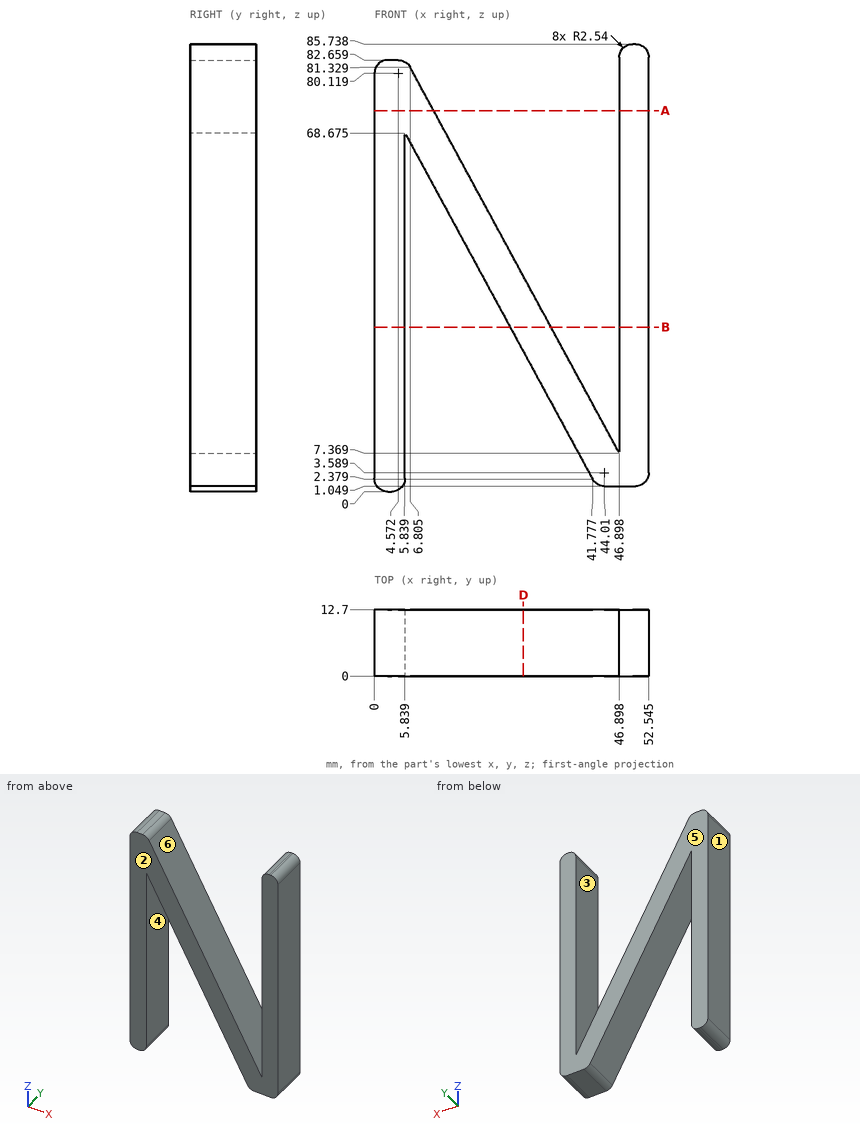
Check sheet for the drawn part. Datum: minimum x, y, z corner. Units: mm. A direction names the side the tool comes from. Coordinates: 2 decimals unless noted, no trailing zeros. Order: outer loops, then holes, each group sorted by start corner. A loop starts at its lowest first (then second) coordinate and runs counter-clockwise, first axis right, second up. Notation, with made-up numbers: (-14.75, 30.5) -> (37.25, 30.5) arc R31 ccw to (37.25, 63.5) -> close; hole circle Ø11 at (18.5, -31.75). An arc over 180 degrees is marked (long way). Write each question's results on one line, items separated by ' | '. Start each with the question number.
1) Material ranges on line 1 along X through (y, z) = (10.5, 45.5) (1 decimal); line 2 along X through (y, z) = (7, 15.5) (1 decimal); line 3 along X through (y, z) = (9.25, 5.5) (1 decimal), recorded low to high.
2) Depth check by flat-ended pin: pin 1 (5 mm diameter, centred on x = 40.5, y = 7.5, fed in from +Z) (1 decimal); pin 2 (5 mm diameter, centred on x = 46.5, y = 5, fed in from -Z); pin 3 (2 mm diameter, centred on x = 38.5, y = 10.5, fed in from +Z) (1 decimal). Enter the tip coordinate at first touch or a pass-through.
3) Section check B-B (z = 31.5). Enter the section's corners in (x, y) (1 decimal).
4) Section check A-A (z = 73). Enter the section's corners in (x, y) (1 decimal).
5) Set-up check for the marked faces 4, 5 and 6: record each of +Z, -Z, +X, -X, +Y, -Y from which the full face is reachable in a straight line by a thin tool's end or side.
6) Draft check along X on the marked faces 1, 2 and 3. Enter one of: pulls with the +X half, pulls with the -X half, needs draft (parallel to the pull), parting line crosses it, or undercut.
7) Section check D-D (x = 28.5). Enter the section's corners in (y, z).
Checked values:
1) line 1: 0 to 5.8, 18.4 to 26.2, 46.9 to 52.5 | line 2: 0 to 5.8, 34.7 to 42.5, 46.9 to 52.5 | line 3: 0 to 5.8, 40.1 to 52.5
2) pin 1: z = 23.8 | pin 2: z = 1.05 | pin 3: z = 24.7
3) outline: (0, 0) -> (5.8, 0) -> (5.8, 12.7) -> (0, 12.7) -> close; (26, 0) -> (33.8, 0) -> (33.8, 12.7) -> (26, 12.7) -> close; (46.9, 0) -> (52.5, 0) -> (52.5, 12.7) -> (46.9, 12.7) -> close
4) outline: (0, 0) -> (11.3, 0) -> (11.3, 12.7) -> (0, 12.7) -> close; (46.9, 0) -> (52.5, 0) -> (52.5, 12.7) -> (46.9, 12.7) -> close
5) face 4: -Z, +Y, -Y | face 5: +Z, -Z, +X, -X, +Y | face 6: +Z, +Y, -Y
6) face 1: pulls with the -X half | face 2: needs draft | face 3: undercut
7) outline: (0, 26.87) -> (12.7, 26.87) -> (12.7, 41.31) -> (0, 41.31) -> close
